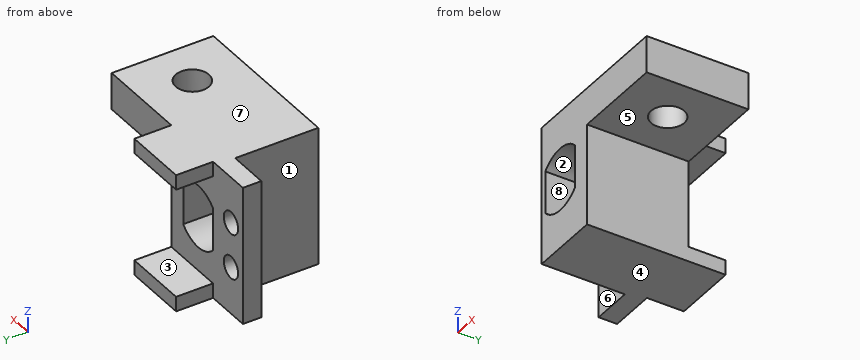
from build123d import *

# Parameters (mm, degrees)
BOSS_EXTRUDE1_DEPTH = 2.54
CUT_EXTRUDE1_DEPTH  = 23.876
SKETCH3_R           = 1.524
CUT_EXTRUDE2_DEPTH  = 2.54
SKETCH4_W           = 8.89
SKETCH4_H           = 2.032
BOSS_EXTRUDE2_DEPTH = 5.08
SKETCH5_W           = 12.7
SKETCH5_H           = 5.08
BOSS_EXTRUDE3_DEPTH = 11.43
SKETCH6_R           = 2.286
CUT_EXTRUDE3_DEPTH  = 11.43
SKETCH7_W           = 9.652
SKETCH7_H           = 19.05
BOSS_EXTRUDE4_DEPTH = 11.43
CUT_EXTRUDE4_DEPTH  = 25.4


with BuildPart() as part:
    # Sketch1 → Boss-Extrude1 (new body)
    with BuildSketch(Plane(origin=(0, 0, 0), x_dir=(1, 0, 0), z_dir=(0, 1, 0))):
        Polygon((0, 0), (12.7, 0), (12.7, -5.08), (-15.24, -5.08), (-15.24, 13.97), (0, 13.97), align=None)
    extrude(amount=BOSS_EXTRUDE1_DEPTH)

    # Sketch2 → Cut-Extrude1 (cut)
    with BuildSketch(Plane(origin=(0, 2.54, 0), x_dir=(1, 0, 0), z_dir=(0, 1, 0))):
        with BuildLine():
            Line((-8.89, 1.45498347), (-8.89, 7.30801653))
            ThreePointArc((-8.89, 7.30801653), (-5.715, 8.6995), (-2.54, 7.30801653))
            Line((-2.54, 7.30801653), (-2.54, 1.45498347))
            ThreePointArc((-2.54, 1.45498347), (-5.715, 0.0635), (-8.89, 1.45498347))
        make_face()
    extrude(amount=-CUT_EXTRUDE1_DEPTH, mode=Mode.SUBTRACT)

    # Sketch3 → Cut-Extrude2 (cut)
    with BuildSketch(Plane(origin=(0, 2.54, 0), x_dir=(1, 0, 0), z_dir=(0, 1, 0))):
        with Locations(Location((-12.7, 1.27, 0), (0, 0, 270))):
            Circle(SKETCH3_R)
        with Locations(Location((-12.7, 7.493, 0), (0, 0, 90))):
            Circle(SKETCH3_R)
    extrude(amount=-CUT_EXTRUDE2_DEPTH, mode=Mode.SUBTRACT)

    # Sketch4 → Boss-Extrude2 (add)
    with BuildSketch(Plane(origin=(0, 2.54, 0), x_dir=(1, 0, 0), z_dir=(0, 1, 0))):
        with Locations((-4.445, 12.954)):
            Rectangle(SKETCH4_W, SKETCH4_H)
        with Locations((-4.445, -4.064)):
            Rectangle(SKETCH4_W, SKETCH4_H)
    extrude(amount=BOSS_EXTRUDE2_DEPTH)

    # Sketch5 → Boss-Extrude3 (add)
    with BuildSketch(Plane.XZ):
        with Locations((6.35, 2.54)):
            Rectangle(SKETCH5_W, SKETCH5_H)
    extrude(amount=BOSS_EXTRUDE3_DEPTH)

    # Sketch6 → Cut-Extrude3 (cut)
    with BuildSketch(Plane(origin=(0, 0, 0), x_dir=(-1, 0, 0), z_dir=(0, 0, -1))):
        with Locations((-6.35, -4.445)):
            Circle(SKETCH6_R)
    extrude(amount=-CUT_EXTRUDE3_DEPTH, mode=Mode.SUBTRACT)

    # Sketch7 → Boss-Extrude4 (add)
    with BuildSketch(Plane.XZ):
        with Locations((-4.826, -4.445)):
            Rectangle(SKETCH7_W, SKETCH7_H)
    extrude(amount=BOSS_EXTRUDE4_DEPTH)

    # Sketch2_3 → Cut-Extrude4 (cut)
    with BuildSketch(Plane(origin=(0, 2.54, 0), x_dir=(1, 0, 0), z_dir=(0, 1, 0))):
        with BuildLine():
            Line((-8.89, 1.45498347), (-8.89, 7.30801653))
            ThreePointArc((-8.89, 7.30801653), (-5.715, 8.6995), (-2.54, 7.30801653))
            Line((-2.54, 7.30801653), (-2.54, 1.45498347))
            ThreePointArc((-2.54, 1.45498347), (-5.715, 0.0635), (-8.89, 1.45498347))
        make_face()
    extrude(amount=-CUT_EXTRUDE4_DEPTH, mode=Mode.SUBTRACT)


solid = part.part
Work out the finished part from the listing and answer in its coordinate system (mm). Face numbers are marked on the shaded views. A direction names the side the tool comes from. Round coordinates to 2 decimals unless told otherwise and drop trailing zeros. Write each loop counter-clockwise with the first axis right and the second up, starting at its lowest first coordinate (ties: lowest second). Pieces come first, ordered by that corner, then holes. Notation, with made-up numbers: (84, -17) -> (103, -17) arc R6 cw to (103, -9) -> close; hole circle Ø1 at (-8.75, 6). An arc over 180 degrees is marked (long way). Answer as CSV lines item,"result". Start each with the question number.
(1) Find the intervals of material crossed by probe 1 along X at (y, z) = (1.9, -1.27); probe 2 along Z at (x, y) = (-1, 3.25); probe 3 along Y at (x, z) = (6.35, 1.3), in increasing order.
(2) A tool of negligible diameter and unlimited length cuts with its end or side. For the marked faces 1, 2, 3, 4 and 5, from which of +Z, -Z, +X, -X, +Y, -Y can it reach the whole face along a straight path? Write none if from no direction.
(3) The part is cut by section B-B, the plane x = 6.35. Give the vertices of the cut face in (y, z), then the cut area to 3 significant figures.
(4) The part is cut by section A-A, the plane y = 5. Give the vertices of the cut face in (x, z).
(5) The part is cut by section D-D, the plane x = -12.7. Give the vertices of the cut face in (y, z), then the cut area to 3 significant figures.
(6) The part is cut by section C-C, the plane y = -8.5. Give the vertices of the cut face in (x, z) (1 decimal).
(7) Each of these flat-tipped pins is pushed along its axis until it touches: pin 1 (6.5 mm diameter, centred on y = -5.5, z = -3, fed in from -X); pin 2 (1 mm diameter, centred on y = 4.5, z = -13, fed in from -X); pin 3 (10 mm diameter, centred on x = 8, y = -6, fed in from -Z); pin 4 (11 mm diameter, centred on y = -3.5, z = -4, fed in from +X). Where does it stop, or does it pass through?
(8) The mould has two halves that part along Z. Classify the marked faces 6, 7 and 8: +Z half, -Z half, draft (parallel to the pull), parting line (faces both ways), or undercut.
Output values:
1,probe 1,"x = -15.24 to -14.22, -11.18 to -8.71, -2.72 to 0"
1,probe 2,"z = -13.97 to -11.94, 3.05 to 5.08"
1,probe 3,"y = -11.43 to -6.73, -2.16 to 2.54"
2,face 1,"+Z, -Z, -X, -Y"
2,face 2,"+Y, -Y"
2,face 3,"+X, -X, +Y"
2,face 4,"-Z, +X, -X, +Y, -Y"
2,face 5,"-Z, +X, +Y, -Y"
3,outline,"(-11.43, 0) -> (-6.73, 0) -> (-6.73, 5.08) -> (-11.43, 5.08) -> close; (-2.16, 0) -> (2.54, 0) -> (2.54, 5.08) -> (-2.16, 5.08) -> close"
3,area,"47.7 mm²"
4,outline,"(-8.89, -13.97) -> (0, -13.97) -> (0, -11.94) -> (-8.89, -11.94) -> close; (-8.89, 3.05) -> (0, 3.05) -> (0, 5.08) -> (-8.89, 5.08) -> close"
5,outline,"(0, -13.97) -> (2.54, -13.97) -> (2.54, -9.02) -> (0, -9.02) -> close; (0, -5.97) -> (2.54, -5.97) -> (2.54, -2.79) -> (0, -2.79) -> close; (0, 0.25) -> (2.54, 0.25) -> (2.54, 5.08) -> (0, 5.08) -> close"
5,area,"32.9 mm²"
6,outline,"(-9.7, -14) -> (0, -14) -> (0, 0) -> (12.7, 0) -> (12.7, 5.1) -> (-9.7, 5.1) -> close; hole (-8.9, -7.3) arc R4.3 ccw to (-2.5, -7.3) -> (-2.5, -1.5) arc R4.3 ccw to (-8.9, -1.5) -> close"
7,pin 1,"stops at x = -9.65"
7,pin 2,"stops at x = -8.89"
7,pin 3,"stops at z = 0"
7,pin 4,"stops at x = 12.7"
8,face 6,"draft"
8,face 7,"+Z half"
8,face 8,"undercut"
